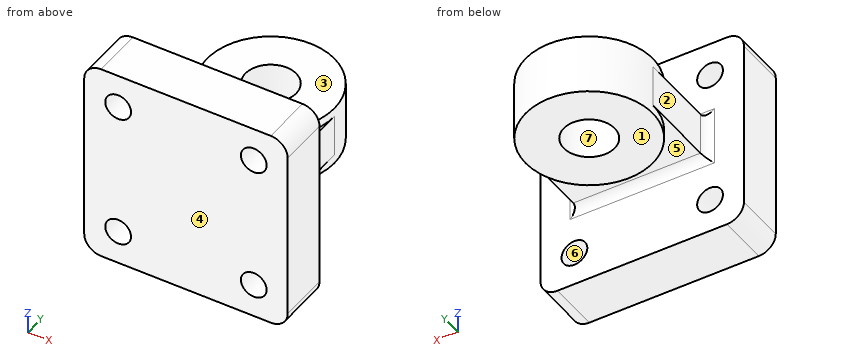
```python
from build123d import *

# Parameters (mm, degrees)
SKETCH1_W           = 76.2
SKETCH1_H           = 76.2
SKETCH1_R           = 4.826
BOSS_EXTRUDE1_DEPTH = 19.05
BOSS_EXTRUDE4_DEPTH = 7.874
SKETCH2_5_R         = 23.8125
SKETCH2_5_R_2       = 9.525
BOSS_EXTRUDE5_DEPTH = 11.176
FILLET1_R           = 3.175
FILLET2_R           = 6.35


with BuildPart() as part:
    # Sketch1 → Boss-Extrude1 (new body)
    with BuildSketch(Plane(origin=(0, 0, 0), x_dir=(1, 0, 0), z_dir=(0, 1, 0))):
        with Locations((38.1, -38.1)):
            Rectangle(SKETCH1_W, SKETCH1_H)
        with Locations((63.5, -63.5)):
            Circle(SKETCH1_R, mode=Mode.SUBTRACT)
        with Locations((12.7, -63.5)):
            Circle(SKETCH1_R, mode=Mode.SUBTRACT)
        with Locations((63.5, -12.7)):
            Circle(SKETCH1_R, mode=Mode.SUBTRACT)
        with Locations((12.7, -12.7)):
            Circle(SKETCH1_R, mode=Mode.SUBTRACT)
    extrude(amount=BOSS_EXTRUDE1_DEPTH)

    # Sketch2 → Boss-Extrude4 (add, symmetric)
    with BuildSketch(Plane.XY.offset(38.1)):
        with BuildLine():
            ThreePointArc((61.9125, 50.8), (38.1, 26.9875), (14.2875, 50.8))
            Line((14.2875, 50.8), (14.2875, 19.05))
            Line((14.2875, 19.05), (61.9125, 19.05))
            Line((61.9125, 19.05), (61.9125, 50.8))
        make_face()
    extrude(amount=BOSS_EXTRUDE4_DEPTH, both=True)

    # Sketch2_5 → Boss-Extrude5 (add, symmetric)
    with BuildSketch(Plane.XY.offset(38.1)):
        with Locations((38.1, 50.8)):
            Circle(SKETCH2_5_R)
        with Locations((38.1, 50.8)):
            Circle(SKETCH2_5_R_2, mode=Mode.SUBTRACT)
    extrude(amount=BOSS_EXTRUDE5_DEPTH, both=True)

    # Fillet1
    fillet1_edges = [part.edges().sort_by_distance(p)[0] for p in [
        (38.1, 19.05, 30.226),
        (14.2875, 19.05, 38.1),
        (61.9125, 19.05, 38.1),
        (38.1, 19.05, 45.974),
    ]]
    fillet(fillet1_edges, radius=FILLET1_R)

    # Fillet2
    fillet2_edges = [part.edges().sort_by_distance(p)[0] for p in [
        (0, 9.525, 0),
        (76.2, 9.525, 0),
        (76.2, 9.525, 76.2),
        (0, 9.525, 76.2),
    ]]
    fillet(fillet2_edges, radius=FILLET2_R)


solid = part.part
```
CAD build for the part. Positions are in the model's coordinates, mm. Face numbers are marked on the shaded views. A direction names the side the tool comes from. Give positions to 0.01 mm unless a question says otherwise; leave off trailing zeros. Write each loop counter-clockwise with the first axis right and the second up, starting at its lowest first coordinate (ties: lowest second). Pieces come first, ordered by that corner, then holes. Notation, with made-up numbers: M 48.5,-23 L 96.5,-23 A29 cw 96.5,14 Z; hole C 55,1 d9. An arc over 180 degrees is marked long. Return JSON: item names as keys, results as strings. Group by question number.
(1) 3-axis set-ups, long thin cutter, end or side, ignore diameter. For the marked faces 1, 2 and 3: which of +Z, -Z, +X, -X, +Y, -Y reach the whole face in a straight line?
(2) Band-saw the part on C-C (y = 59). Give the cut face in (x, z), and give its area (3 significant figures).
(3) Mould opens along Y. For the marked faces 4, 5, 6 and 7 say: pulls with the +Y half, pulls with the -Y half, needs draft (parallel to the pull), parting line crosses it, or undercut.
(4) Drill centre lines: L1, parallel to X at y = 7.25, z = 63.5; L2, parallel to Y at x = 38.1, z = 35 (1 decimal). Where is each one in solid material? Low to high. Write a range as [from, to].
(5) Band-saw the part on B-B (z = 12.7). Give the cut face in (x, y), and give its area (3 significant figures).
(6) Band-saw the part on D-D (x = 9.5). Give the cut face in (y, z), and give its area (3 significant figures).
(7) Flat gauge pins, fed straight in: pin 1 Ø14.5 at (x, y) = (48.5, 54.5) entering from +Z; pin 2 Ø7.5 at (x, z) = (12.7, 63.5) entering from -Y; pin 3 Ø2 at (y, z) = (63, 32) entering from -X; pin 4 Ø6 at (x, z) = (55, 38.5) entering from +Y. Where does each tip first touch, or does it go through?
Entries:
{
 "1": {"face 1": "-Z, +X, -X, +Y", "face 2": "+Z, -Z, -X, +Y", "face 3": "+Z, +X, -X, +Y"},
 "2": {"outline": "M 15.74,26.92 L 33.25,26.92 L 33.25,49.28 L 15.74,49.28 Z; M 42.95,26.92 L 60.46,26.92 L 60.46,49.28 L 42.95,49.28 Z", "area": "783 mm^2"},
 "3": {"face 4": "pulls with the -Y half", "face 5": "undercut", "face 6": "needs draft", "face 7": "undercut"},
 "4": {"L1": "x = [0, 7.87], [17.53, 58.67], [68.33, 76.2]", "L2": "y = [0, 41.3], [60.3, 74.6]"},
 "5": {"outline": "M 0,0 L 7.87,0 L 7.87,19.05 L 0,19.05 Z; M 17.53,0 L 58.67,0 L 58.67,19.05 L 17.53,19.05 Z; M 68.33,0 L 76.2,0 L 76.2,19.05 L 68.33,19.05 Z", "area": "1,080 mm^2"},
 "6": {"outline": "M 0,0 L 19.05,0 L 19.05,9.09 L 0,9.09 Z; M 0,16.31 L 19.05,16.31 L 19.05,59.89 L 0,59.89 Z; M 0,67.11 L 19.05,67.11 L 19.05,76.2 L 0,76.2 Z", "area": "1,180 mm^2"},
 "7": {"pin 1": "stops at z = 49.28", "pin 2": "passes through", "pin 3": "stops at x = 17.09", "pin 4": "stops at y = 70.13"}
}
